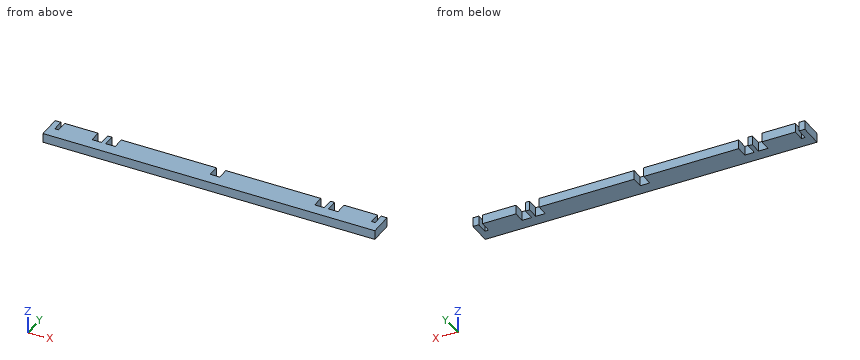
Autodesk Inventor part; units mm, degrees
ref_plane "YZ Plane" through (0, 0, 0) normal (1, 0, 0) x (0, 1, 0)
ref_plane "XZ Plane" through (0, 0, 0) normal (0, 1, 0) x (-1, 0, 0)
ref_plane "XY Plane" through (0, 0, 0) normal (0, 0, 1) x (1, 0, 0)
sketch "Sketch1" plane through (0, 0, 0) normal (0, 0, 1) x (1, 0, 0)
  line L0 (0, 0) -> (143.2, 0)
  line L1 (143.2, 0) -> (143.2, 20)
  line L2 (143.2, 20) -> (138.2, 20)
  line L3 (138.2, 20) -> (138.2, 10)
  line L4 (138.2, 10) -> (135, 10)
  line L5 (135, 10) -> (135, 20)
  line L6 (135, 20) -> (106.1, 20)
  line L7 (106.1, 20) -> (106.1, 10)
  line L8 (106.1, 10) -> (97.9, 10)
  line L9 (97.9, 10) -> (97.9, 20)
  line L10 (97.9, 20) -> (94.3, 20)
  line L11 (94.3, 20) -> (94.3, 10)
  line L12 (94.3, 10) -> (86.1, 10)
  line L13 (86.1, 10) -> (86.1, 20)
  line L14 (86.1, 20) -> (4.1, 20)
  line L15 (4.1, 20) -> (4.1, 10)
  line L16 (4.1, 10) -> (0, 10)
  line L17 (0, 50) -> (0, 0)
  line L18 (0, 0) -> (-143.2, 0)
  line L19 (-143.2, 0) -> (-143.2, 20)
  line L20 (-143.2, 20) -> (-138.2, 20)
  line L21 (-138.2, 20) -> (-138.2, 10)
  line L22 (-138.2, 10) -> (-135, 10)
  line L23 (-135, 10) -> (-135, 20)
  line L24 (-135, 20) -> (-106.1, 20)
  line L25 (-106.1, 20) -> (-106.1, 10)
  line L26 (-106.1, 10) -> (-97.9, 10)
  line L27 (-97.9, 10) -> (-97.9, 20)
  line L28 (-97.9, 20) -> (-94.3, 20)
  line L29 (-94.3, 20) -> (-94.3, 10)
  line L30 (-94.3, 10) -> (-86.1, 10)
  line L31 (-86.1, 10) -> (-86.1, 20)
  line L32 (-86.1, 20) -> (-4.1, 20)
  line L33 (-4.1, 20) -> (-4.1, 10)
  line L34 (-4.1, 10) -> (0, 10)
  dimension "d4" = 3.2
  dimension "d5" = 20
  dimension "d6" = 10
  dimension "d7" = 0
  dimension "d8" = 82
  dimension "d9" = 0
  dimension "d10" = 135
  dimension "d11" = 20
  dimension "d12" = 5
  dimension "d13" = 8.2
  dimension "d14" = 8.2
  dimension "d15" = 4.1
  dimension "d16" = 50
extrude "Extrusion1" add sketch "Sketch1" along normal blind 8
properties part number "brace"
Here's how the part is built. I have some questions about the finished solid (model axes, mm). Coordinates: 2 decimals unless noted, no trailing zeros. Write each loop counter-clockwise with the first axis right and the second up, starting at its lowest first coordinate (ties: lowest second). Pieces come first, ordered by that corner, then holes. Notation, with made-up numbers: (16.25, -25) -> (56.25, -25) arc R7 ccw to (56.25, -16) -> close; hole circle Ø7 at (28, 84.5). An arc over 180 degrees is marked (long way). Use a Markdown table: item, result. Add a question column.
(1) I'm going to push a flat-ended pin straight in: P1, Ø4, axis at x = 103, z = 5, coming from the +Y side. Where does the tip first touch, or does it pass through?
(2) Please list where this line runs through material, in increasing order: line 1 (Y direction, x = -87.5, z = 1).
(3) If we section it at C-C, the plane x = 89: Write out the boundary of the cut face in (y, z), and give its area (3 significant figures).
(4) If we section it at A-A, the plane y = 16.75: State how many separate pieces and enclosed holes the cut face has, and give its area (3 significant figures).
Outcome:
| question | item | result |
|---|---|---|
| 1 | P1 | stops at y = 10 |
| 2 | line 1 | y = 0 to 10 |
| 3 | outline | (0, 0) -> (10, 0) -> (10, 8) -> (0, 8) -> close |
| 3 | area | 80.0 mm^2 |
| 4 | separate pieces | 8 |
| 4 | enclosed holes | 0 |
| 4 | area | 1,910 mm^2 |
